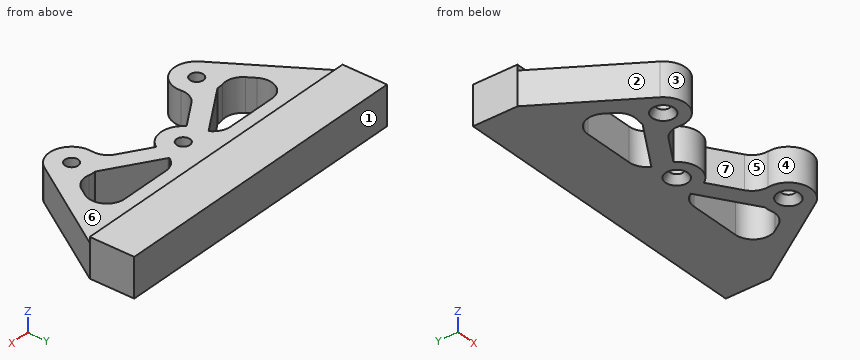
```python
from build123d import *

# Parameters (mm, degrees)
F1_DEPTH       = 9.525
F2_T1_DEPTH    = 9.525
F3_W           = 88.9
F3_H           = 12.7
F4_DEPTH       = 1.5875
F6_D           = 3.81
F6_CSINK_D     = 6.35
F6_CSINK_ANGLE = 60


# Not quite as in the source:
# - a fillet or chamfer that OpenCascade refuses, or shapes differently, is made with other operations: its cross-section is extruded or revolved along the edge and cut away or added


with BuildPart() as f1:
    # F0 (on Top) → F1 (new body)
    with BuildSketch(Plane.XY):
        with BuildLine():
            Line((-16.6466649714, -10.6111378352), (-5.3546547037, -3.4132349764))
            ThreePointArc((-5.3546547037, -3.4132349764), (0, -6.35), (5.3546547037, -3.4132349764))
            Line((5.3546547037, -3.4132349764), (16.6466649714, -10.6111378352))
            ThreePointArc((16.6466649714, -10.6111378352), (18.5880846986, -19.3790275153), (27.3559743788, -17.437607788))
            Line((27.3559743788, -17.437607788), (44.45, 9.3793577389))
            Line((44.45, 9.3793577389), (44.45, 22.0793577389))
            Line((44.45, 22.0793577389), (-44.45, 22.0793577389))
            Line((-44.45, 22.0793577389), (-44.45, 9.3793577389))
            Line((-44.45, 9.3793577389), (-27.3559743788, -17.437607788))
            ThreePointArc((-27.3559743788, -17.437607788), (-18.5880846986, -19.3790275153), (-16.6466649714, -10.6111378352))
        make_face()
        with BuildLine():
            Line((-5.9433808033, 2.2357827771), (-21.519114834, -7.6927080628))
            ThreePointArc((-21.519114834, -7.6927080628), (-24.1573435523, -8.0515961507), (-26.4165242416, -9.4605510978))
            Line((-26.4165242416, -9.4605510978), (-35.1875477179, 4.2993577389))
            Line((-35.1875477179, 4.2993577389), (-4.6731170575, 4.2993577389))
            ThreePointArc((-4.6731170575, 4.2993577389), (-5.4075957794, 3.3287246638), (-5.9433808033, 2.2357827771))
        make_face(mode=Mode.SUBTRACT)
        with BuildLine():
            ThreePointArc((5.9433808033, 2.2357827771), (5.4075957794, 3.3287246638), (4.6731170575, 4.2993577389))
            Line((4.6731170575, 4.2993577389), (35.1875477179, 4.2993577389))
            Line((35.1875477179, 4.2993577389), (26.4165242416, -9.4605510978))
            ThreePointArc((26.4165242416, -9.4605510978), (24.1573435523, -8.0515961507), (21.519114834, -7.6927080628))
            Line((21.519114834, -7.6927080628), (5.9433808033, 2.2357827771))
        make_face(mode=Mode.SUBTRACT)
    extrude(amount=F1_DEPTH)

    # F2: fillet of radius 5.08 on 10 edges, made by hand

    # F2_s2 → F2_t1 (join)
    with BuildSketch(Plane.XY):
        with BuildLine():
            ThreePointArc((25.9250954358, 4.2993577389), (30.3791827129, 1.6622057751), (30.2088191987, -3.5112302422))
            Line((30.2088191987, -3.5112302422), (35.1875477179, 4.2993577389))
            Line((35.1875477179, 4.2993577389), (25.9250954358, 4.2993577389))
        make_face()
        with BuildLine():
            ThreePointArc((28.86470245, -5.6198694424), (26.5021187872, -7.5920062794), (23.4344635706, -7.8382109503))
            ThreePointArc((23.4344635706, -7.8382109503), (25.0359187955, -8.4464064996), (26.4165242416, -9.4605510978))
            Line((26.4165242416, -9.4605510978), (28.86470245, -5.6198694424))
        make_face()
        with BuildLine():
            ThreePointArc((6.3351726778, -0.433690145), (7.9360436505, 2.9321004414), (11.4033108201, 4.2993577389))
            Line((11.4033108201, 4.2993577389), (4.6731170575, 4.2993577389))
            ThreePointArc((4.6731170575, 4.2993577389), (5.9913309283, 2.1039139022), (6.3351726778, -0.433690145))
        make_face()
        with BuildLine():
            ThreePointArc((5.4870763048, 3.1960121441), (6.2133994477, 2.2333964199), (7.1461493675, 1.4690980964))
            Line((7.1461493675, 1.4690980964), (5.9433808033, 2.2357827771))
            ThreePointArc((5.9433808033, 2.2357827771), (5.7353594076, 2.7254637156), (5.4870763048, 3.1960121441))
        make_face()
        with BuildLine():
            ThreePointArc((-7.1461493675, 1.4690980964), (-6.2133994477, 2.2333964199), (-5.4870763048, 3.1960121441))
            ThreePointArc((-5.4870763048, 3.1960121441), (-5.7353594076, 2.7254637156), (-5.9433808033, 2.2357827771))
            Line((-5.9433808033, 2.2357827771), (-7.1461493675, 1.4690980964))
        make_face()
        with BuildLine():
            ThreePointArc((-11.4033108201, 4.2993577389), (-7.9360436505, 2.9321004414), (-6.3351726778, -0.433690145))
            ThreePointArc((-6.3351726778, -0.433690145), (-5.9913309283, 2.1039139022), (-4.6731170575, 4.2993577389))
            Line((-4.6731170575, 4.2993577389), (-11.4033108201, 4.2993577389))
        make_face()
        with BuildLine():
            ThreePointArc((-23.4344635706, -7.8382109503), (-26.5021187872, -7.5920062794), (-28.86470245, -5.6198694424))
            Line((-28.86470245, -5.6198694424), (-26.4165242416, -9.4605510978))
            ThreePointArc((-26.4165242416, -9.4605510978), (-25.0359187955, -8.4464064996), (-23.4344635706, -7.8382109503))
        make_face()
        with BuildLine():
            ThreePointArc((-30.2088191987, -3.5112302422), (-30.3791827129, 1.6622057751), (-25.9250954358, 4.2993577389))
            Line((-25.9250954358, 4.2993577389), (-35.1875477179, 4.2993577389))
            Line((-35.1875477179, 4.2993577389), (-30.2088191987, -3.5112302422))
        make_face()
        with BuildLine():
            ThreePointArc((-15.6875923106, -13.3466215538), (-15.2148846453, -10.6031015998), (-13.3671984002, -8.5206967846))
            Line((-13.3671984002, -8.5206967846), (-16.6466649714, -10.6111378352))
            ThreePointArc((-16.6466649714, -10.6111378352), (-16.0089492913, -11.9234213166), (-15.6875923106, -13.3466215538))
        make_face()
        with BuildLine():
            ThreePointArc((13.3671984002, -8.5206967846), (15.2148846453, -10.6031015998), (15.6875923106, -13.3466215538))
            ThreePointArc((15.6875923106, -13.3466215538), (16.0089492913, -11.9234213166), (16.6466649714, -10.6111378352))
            Line((16.6466649714, -10.6111378352), (13.3671984002, -8.5206967846))
        make_face()
    extrude(amount=F2_T1_DEPTH)

    # F3 (on face) → F4 (join)
    with BuildSketch(Plane.XY.offset(9.525)):
        with Locations((0, 15.7293577389)):
            Rectangle(F3_W, F3_H)
    extrude(amount=F4_DEPTH)

    # F6 (through all)
    with Locations(Plane(origin=(0, 0, 0), x_dir=(1, 0, 0), z_dir=(0, 0, -1))):
        with Locations((0, 0), (-22.0013196751, 14.0243728116), (22.0013196751, 14.0243728116)):
            CounterSinkHole(F6_D / 2, F6_CSINK_D / 2, counter_sink_angle=F6_CSINK_ANGLE)


solid = f1.part
```
The model under review builds one solid part; all positions refer to its coordinate system, in mm. Face numbers are marked on the shaded views. A direction names the side the tool comes from. Round coordinates to 2 decimals unless told otherwise and drop trailing zeros. Loops run counter-clockwise (first coordinate to the right, second up) from the corner with the lowest first, then second, coordinate; pieces in that order, holes last. Notation, with made-up numbers: M 65.5,85 L 96.5,85 A6 cw 96.5,90 Z; hole C 48,43 d4. An arc over 180 degrees is marked long. Write item = value, one per line.
Item 1: Take a section at B-B on y = 0. Write out the cut boundary in (x, z) (3 decimals), then the cut area to 3 significant figures.
Return value:
outline = M -38.471,0 L -30.945,0 L -30.945,9.525 L -38.471,9.525 Z; M -9.451,0 L -3.175,0 L -1.905,2.2 L -1.905,9.525 L -9.451,9.525 Z; M 1.905,2.2 L 3.175,0 L 9.451,0 L 9.451,9.525 L 1.905,9.525 Z; M 30.945,0 L 38.471,0 L 38.471,9.525 L 30.945,9.525 Z
area = 284 mm2
Item 2: The part is to be moulded in two halves that separate along X. For the marked faces 1, 2, 3 and 4, say which applies: released by +X, released by -X, zero draft, split by the parting line, or undercut.
Return value:
face_1 = zero draft
face_2 = released by -X
face_3 = undercut
face_4 = undercut
Item 3: Insertion check: P1, Ø2.5, axis at x = 0, y = 0, coming from the -Z side; P2, Ø4, axis at y = -5, z = 6, coming from the -X side; P3, Ø15, axis at x = 2.5, y = 1.5, coming from the +Z side (3 decimals); P4, Ø5, axis at x = 16, z = 6.5, coming from the -Y side. Each pin has a flat end and moves straight along its axis. Give the tip position at first contact, or say it passes through.
Return value:
P1 = through
P2 = -36.56
P3 = 9.525
P4 = -19.32
Item 4: Take a section at C-C on z = 5.25. State how many separate pieces and enclosed holes the cut face has, then the cut area to 3 significant figures.
Return value:
separate_pieces = 1
enclosed_holes = 5
area = 2,310 mm2
Item 5: For line 1 (Y direction, x = -23.5, z = 0.75); line 2 (Y direction, x = 0, z = 4.75) (3 decimals); line 3 (Y direction, x = 22.5, z = 3), list the stretches that pass through material, from the lowest coordinate up. Write a range as [from, to].
Return value:
line_1 = [-20.19, -16.32], [-11.73, -7.85], [4.3, 22.08]
line_2 = [-6.35, -1.905], [1.905, 22.079]
line_3 = [-20.35, -15.86], [-12.19, -7.69], [4.3, 22.08]
Item 6: Machinability: for the marked faces 5, 6 and 7, which of the approach directions +Z, -Z, +X, -X, +Y, -Y give a long, thin tool a straight path to every point of the face, cutting with its end or side? Answer none if there is none.
Return value:
face_5 = +Z, -Z
face_6 = +Z, +X, -X, -Y
face_7 = +Z, -Z, -Y
